Design review of the part built by this model. Coordinates are the model's own, in mm. Face numbers are marked on the shaded views. A direction names the side the tool comes from. Give positions to 0.01 mm unless a question says otherwise; leave off trailing zeros. Loops run counter-clockwise (first coordinate to the right, second up) from the corner with the lowest first, then second, coordinate; pieces in that order, holes last. Notation, with made-up numbers: (53.25, 57.5) -> (103.25, 57.5) arc R18 ccw to (103.25, 91.5) -> close; hole circle Ø9 at (3, 82). An arc over 180 degrees is marked (long way). Answer in a Markdown table with one row per item. Add a question column.
(1) For line 1 (Y direction, x = 0, z = 10.25); line 2 (Y direction, x = 0, z = 8.75); line 3 (Z direction, x = 5, y = 19), list the stretches that pass through material, from the lowest coordinate up.
(2) Consider section B-B on x = 0. Count the separate pieces of the cut face and the enclosed holes in it, then the cut area to 3 significant figures.
(3) Draft analysis for pull direction X (two halves, no side actions). For the marked faces 3, 4 and 5, state which applies: +X half, -X half, draft (parallel to the pull), parting line (faces both ways), or undercut.
(4) For pin 1 (5 mm diameter, centred on x = 17.5, z = 6.5, fed in from +Y); pin 2 (4 mm diameter, centred on x = -17, y = 7, fed in from +Z); pin 3 (6 mm diameter, centred on x = 0, y = 0, fed in from -Z); pin 4 (4 mm diameter, centred on x = 9, z = 2, fed in from +Y), all flat-tipped, find the tip position at first contact; note any pin that passes through.
(5) Consider section A-A on y = 0. Write out the cut boundary in (x, z), then the cut area to 3 significant figures.
(6) For the marked faces 1 and 2, list the 3-axis set-ups (+Z, -Z, +X, -X, +Y, -Y) from which the entire face can be reached by the end or side of a thin tool; tool diameter is ignored.
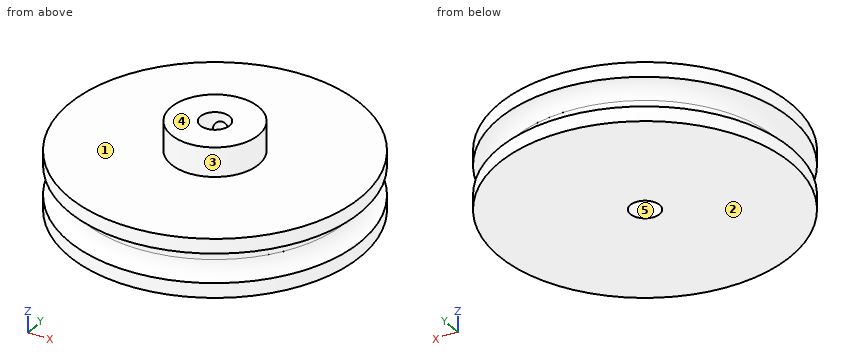
from build123d import *

# Parameters (mm, degrees)
ESQUISSE1_R             = 25
BOSS_EXTRU_1_DEPTH      = 10
ESQUISSE2_R             = 2.5
ESQUISSE5_R             = 7.5
BOSS_EXTRU_3_DEPTH      = 5
ESQUISSE6_R             = 2.5
ENL_V_MAT_EXTRU_2_DEPTH = 39.405728739
TROU_TARAUD_M31_D       = 2.5
TROU_TARAUD_M31_DEPTH   = 8.5
TROU_TARAUD_M31_TIP     = 0.751075774


with BuildPart() as part:
    # Esquisse1 → Boss.-Extru.1 (new body)
    with BuildSketch(Plane.XY):
        Circle(ESQUISSE1_R)
    extrude(amount=BOSS_EXTRU_1_DEPTH)

    # Esquisse2 → Enlèvement de matière-Révolution1 (revolve, cut)
    with BuildSketch(Plane(origin=(0, 0, 0), x_dir=(1, 0, 0), z_dir=(0, 1, 0))):
        with Locations((-25, -5)):
            Circle(ESQUISSE2_R)
    revolve(axis=Axis((0, 0, 0), (0, 0, 1)), mode=Mode.SUBTRACT)

    # Esquisse5 → Boss.-Extru.3 (add)
    with BuildSketch(Plane.XY.offset(10)):
        Circle(ESQUISSE5_R)
    extrude(amount=BOSS_EXTRU_3_DEPTH)

    # Esquisse6 → Enlèv. mat.-Extru.2 (cut, through all)
    with BuildSketch(Plane.XY.offset(15)):
        Circle(ESQUISSE6_R)
    extrude(amount=-ENL_V_MAT_EXTRU_2_DEPTH, mode=Mode.SUBTRACT)

    # Trou taraudé M31
    with Locations(Plane(origin=(-0.924122453, 7.442848762, 12.279526522), x_dir=(0.992379834907, 0.123216327128, 0), z_dir=(-0.123216327128, 0.992379834907, 0))):
        with Locations((0, 0)):
            Hole(TROU_TARAUD_M31_D / 2, depth=TROU_TARAUD_M31_DEPTH)
            with Locations((0, 0, -(TROU_TARAUD_M31_DEPTH + TROU_TARAUD_M31_TIP / 2))):  # 118° drill point
                Cone(0, TROU_TARAUD_M31_D / 2, TROU_TARAUD_M31_TIP, mode=Mode.SUBTRACT)


solid = part.part
Values follow:
| question | item | result |
|---|---|---|
| 1 | line 1 | -7.5 to -2.5, 2.5 to 7.5 |
| 1 | line 2 | -25 to -2.5, 2.5 to 25 |
| 1 | line 3 | 0 to 10 |
| 2 | separate pieces | 3 |
| 2 | enclosed holes | 0 |
| 2 | area | 470 mm2 |
| 3 | face 3 | parting line |
| 3 | face 4 | draft |
| 3 | face 5 | undercut |
| 4 | pin 1 | y = 19.84 |
| 4 | pin 2 | z = 10 |
| 4 | pin 3 | z = 0 |
| 4 | pin 4 | y = 24 |
| 5 | outline | (-25, 0) -> (-2.5, 0) -> (-2.5, 15) -> (-7.5, 15) -> (-7.5, 10) -> (-25, 10) -> (-25, 7.5) arc R2.5 cw to (-25, 2.5) -> close; (2.5, 0) -> (25, 0) -> (25, 2.5) arc R2.5 cw to (25, 7.5) -> (25, 10) -> (7.5, 10) -> (7.5, 15) -> (2.5, 15) -> close |
| 5 | area | 480 mm2 |
| 6 | face 1 | +Z |
| 6 | face 2 | -Z, +X, -X, +Y, -Y |
